```python
from build123d import *

# Parameters (mm, degrees)
BOSS_EXTRUDE1_DEPTH = 6.5
CUT_EXTRUDE1_START  = 11
SKETCH2_R           = 0.8
CUT_EXTRUDE1_DEPTH  = 23
FILLET1_R           = 2
POT_INSERT_DEPTH    = 2.5
POT_START           = 2.5
SKETCH6_R           = 2.75
POT_HOLE_DEPTH      = 1.5


with BuildPart() as part:
    # Sketch1 → Boss-Extrude1 (new body)
    with BuildSketch(Plane.XY):
        with BuildLine():
            Line((3.5, 12), (3.5, 5))
            Line((3.5, 5), (10, 5))
            Line((10, 5), (10, -3))
            Line((10, -3), (3.5, -3))
            Line((3.5, -3), (3.5, -11))
            Line((3.5, -11), (0, -11))
            ThreePointArc((0, -11), (-11.5, 0.5), (0, 12))
            Line((0, 12), (3.5, 12))
        make_face()
    extrude(amount=BOSS_EXTRUDE1_DEPTH)

    # Sketch2 → Cut-Extrude1 (cut, through all)
    with BuildSketch(Plane(origin=(0, 0, 0), x_dir=(1, 0, 0), z_dir=(0, 1, 0)).offset(CUT_EXTRUDE1_START)):
        with Locations((8.5, -4.5)):
            Circle(SKETCH2_R)
        with Locations((5.5, -4.5)):
            Circle(SKETCH2_R)
    extrude(amount=-CUT_EXTRUDE1_DEPTH, mode=Mode.SUBTRACT)

    # Fillet1
    fillet1_edges = [part.edges().sort_by_distance(p)[0] for p in [
        (1.75, 12, 6.5),
        (-11.5, 0.5, 6.5),
        (1.75, -11, 6.5),
    ]]
    fillet(fillet1_edges, radius=FILLET1_R)

    # Sketch5 → Pot Insert (cut)
    with BuildSketch(Plane.XY):
        Polygon((-5.5, -1), (-4, -4), (-4, -5), (0, -5), (4.25, -5), (4.25, -4), (10, -4), (10, 0.5), (10, 5), (4.25, 5), (4.25, 6), (0, 6), (-4, 6), (-4, 5), (-5.5, 2), (-5.5, 0.5), align=None)
    extrude(amount=POT_INSERT_DEPTH, mode=Mode.SUBTRACT)

    # Sketch6 → Pot Hole (cut)
    with BuildSketch(Plane.XY.offset(POT_START)):
        Circle(SKETCH6_R)
    extrude(amount=POT_HOLE_DEPTH, mode=Mode.SUBTRACT)


solid = part.part
```
Design review of the part built by this model. Coordinates are the model's own, in mm. A direction names the side the tool comes from. Coordinates: 2 decimals unless noted, no trailing zeros. Write each loop counter-clockwise with the first axis right and the second up, starting at its lowest first coordinate (ties: lowest second). Pieces come first, ordered by that corner, then holes.
1) Add section A-A (x = 8.5). Write out the cut boundary in (y, z).
2) Add section D-D (x = 1.25). Write out the cut boundary in (y, z), plus the area to 3 significant figures.
3) Mouldability with a two-part tool opening along Z and no side actions: class faces 4 (the flat face through (0, 0, 4)), 5 (the cylindrical face through (4.7, 1.1, 4.5)), 6 (the flat face through (-5.5, 1, 1)), 7 (the flat face through (0, 1, 6.5)) as +Z half, -Z half, draft (parallel to the pull), parting line (faces both ways), or undercut.
4) Insertion check: pin 1 (1.2 mm diameter, centred on y = 0.5, z = 1.5, fed in from +X); pin 2 (1.5 mm diameter, centred on y = 9.5, z = 2, fed in from -X); pin 3 (5.5 mm diameter, centred on x = 5.5, y = -1.5, fed in from -Z). Each pin has a flat end and moves straight along its axis. Give the tip position at first contact, or say it passes through.
5) Add section B-B (y = 0.5). Write out the cut boundary in (x, z), plus the area to 3 significant figures.
6) To check wall thickness, follow L1, parallel to X at y = 0.75, z = 4.5; L2, parallel to Y at x = 0, z = 3.65; L3, parallel to Z at x = 5.5, y = -1. State the ranges of each line that lie inside material, in increasing order.
7) Add section C-C (z = 5). Write out the cut boundary in (x, y).
8) Machinability: for faces 1 (the flat face through (3.5, -7, 3)), 2 (the flat face through (0, 6, 1)), 3 (the flat face through (7, 5, 4)), which of the approach directions +Z, -Z, +X, -X, +Y, -Y give a long, thin tool a straight path to every point of the face, cutting with its end or side? Answer none if there is none.
Check result:
1. outline: (-3, 2.5) - (5, 2.5) - (5, 3.7) - (-3, 3.7) - close; (-3, 5.3) - (5, 5.3) - (5, 6.5) - (-3, 6.5) - close
2. outline: (-11, 0) - (-5, 0) - (-5, 2.5) - (-2.45, 2.5) - (-2.45, 4) - (2.45, 4) - (2.45, 2.5) - (6, 2.5) - (6, 0) - (12, 0) - (12, 4.5) arc R2 ccw to (10, 6.5) - (-9, 6.5) arc R2 ccw to (-11, 4.5) - close
2. area: 113 mm2
3. face 4: -Z half
3. face 5: undercut
3. face 6: draft
3. face 7: +Z half
4. pin 1: stops at x = -5.5
4. pin 2: stops at x = -8.01
4. pin 3: stops at z = 2.5
5. outline: (-11.5, 0) - (-5.5, 0) - (-5.5, 2.5) - (-2.7, 2.5) - (-2.7, 4) - (2.7, 4) - (2.7, 2.5) - (10, 2.5) - (10, 6.5) - (-9.5, 6.5) arc R2 ccw to (-11.5, 4.5) - close; hole circle Ø1.6 at (5.5, 4.5); hole circle Ø1.6 at (8.5, 4.5)
5. area: 88.0 mm2
6. L1: x = -11.5 to 4.7, 6.3 to 7.7, 9.3 to 10
6. L2: y = -11 to -2.75, 2.75 to 12
6. L3: z = 2.5 to 3.7, 5.3 to 6.5
7. outline: (0, -10.94) - (3.5, -10.94) - (3.5, -3) - (4.88, -3) - (4.88, 5) - (3.5, 5) - (3.5, 11.94) - (0, 11.94) arc R11.44 ccw to start; (6.12, -3) - (7.88, -3) - (7.88, 5) - (6.12, 5) - close; (9.12, -3) - (10, -3) - (10, 5) - (9.12, 5) - close
8. face 1: +Z, -Z, +X, -Y
8. face 2: -Z, +X
8. face 3: +Z, -Z, +X, +Y
